Can you work these out from the model? Positions are in its coordinate system, mm. Face numbers are marked on the shaded views. A direction names the side the tool comes from. Give positions to 0.01 mm unless a question says otherwise; leave off trailing zeros. Write each loop counter-clockwise with the first axis right and the second up, starting at its lowest first coordinate (ties: lowest second). Pieces come first, ordered by that corner, then holes. Notation, with made-up numbers: M -5.5,42 L 34.5,42 A21 ccw 34.5,71 Z; hole C 35.25,70.5 d7. An arc over 180 degrees is marked long. Write each question's results on one line, items separated by ' | '.
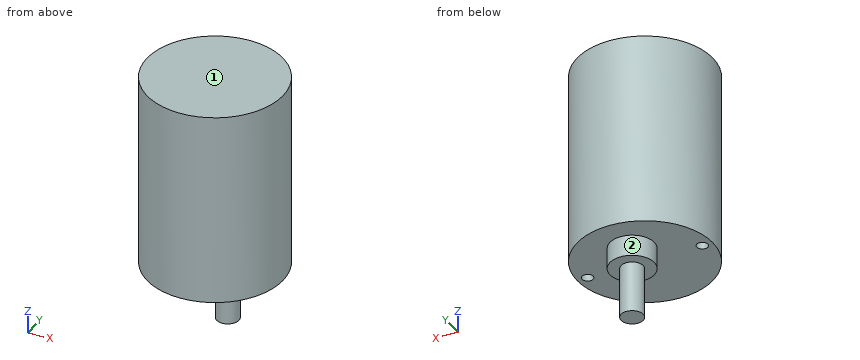
from build123d import *

# Parameters (mm, degrees)
SKETCH_1_R          = 18.35
EXTRUDE_1_DEPTH     = 52.4
SKETCH_1_4_R        = 6
EXTRUDE_2_DEPTH     = 5.7
SKETCH_1_5_R        = 3
EXTRUDE_3_DEPTH     = 19.5
SKETCH_1_6_R        = 1.5
CUT_EXTRUDE_1_DEPTH = 3


with BuildPart() as part:
    # 草图1 → 凸台-拉伸1 (new body)
    with BuildSketch(Plane.XY):
        Circle(SKETCH_1_R)
    extrude(amount=EXTRUDE_1_DEPTH)

    # 草图1<4> → 凸台-拉伸2 (add)
    with BuildSketch(Plane.XY):
        with Locations((0, 6.65)):
            Circle(SKETCH_1_4_R)
    extrude(amount=-EXTRUDE_2_DEPTH)

    # 草图1<5> → 凸台-拉伸3 (add)
    with BuildSketch(Plane.XY):
        with Locations((0, 6.65)):
            Circle(SKETCH_1_5_R)
    extrude(amount=-EXTRUDE_3_DEPTH)

    # 草图1<6> → 切除-拉伸1 (cut)
    with BuildSketch(Plane.XY):
        with Locations((-15.5, 0)):
            Circle(SKETCH_1_6_R)
        with Locations((15.5, 0)):
            Circle(SKETCH_1_6_R)
    extrude(amount=CUT_EXTRUDE_1_DEPTH, mode=Mode.SUBTRACT)


solid = part.part
Item 1: I want a section at B-B, the plane y = 4.5. Please give me the cut outline in (x, z), and give its area (3 significant figures).
Geometry says:
outline: M -17.79,0 L -5.6,0 L -5.6,-5.7 L -2.09,-5.7 L -2.09,-19.5 L 2.09,-19.5 L 2.09,-5.7 L 5.6,-5.7 L 5.6,0 L 17.79,0 L 17.79,52.4 L -17.79,52.4 Z | area: 1,990 mm2
Item 2: If I drill on line 1 (Z direction, x = 3.5, y = 8); line 2 (Z direction, x = -14, y = 8); line 3 (Y direction, x = 15.5, z = 1.9), over which ranges is the centre line in solid material (lowest first)? Write a range as from..to.
Geometry says:
line 1: z = -5.7..52.4 | line 2: z = 0..52.4 | line 3: y = -9.82..-1.5, 1.5..9.82
Item 3: For the marked faces 1 and 2, which set-ups out of +Z, -Z, +X, -X, +Y, -Y let a thin tool reach every point of the face, with its end or its side?
Geometry says:
face 1: +Z, +X, -X, +Y, -Y | face 2: -Z
Item 4: I want a section at D-D, the plane x = 16. Please give me the cut outline in (y, z), and give its area (3 significant figures).
Geometry says:
outline: M -8.98,0 L -1.41,0 L -1.41,3 L 1.41,3 L 1.41,0 L 8.98,0 L 8.98,52.4 L -8.98,52.4 Z | area: 933 mm2
Item 5: I want a section at C-C, the plane z = 17.5. Please give me the cut outline in (x, y).
Geometry says:
outline: C 0,0 d36.7
Item 6: I want a section at A-A, the plane x = 0. Please give me the cut outline in (y, z).
Geometry says:
outline: M -18.35,0 L 0.65,0 L 0.65,-5.7 L 3.65,-5.7 L 3.65,-19.5 L 9.65,-19.5 L 9.65,-5.7 L 12.65,-5.7 L 12.65,0 L 18.35,0 L 18.35,52.4 L -18.35,52.4 Z
Item 7: I'm going to push flat-ended pins straight in: pin 1 (10 mm diameter, centred on x = 13.5, y = -0.5, fed in from -Z); pin 2 (2 mm diameter, centred on x = 5, z = 18, fed in from +Y); pin 3 (1.5 mm diameter, centred on x = -15.5, y = -0.5, fed in from -Z). Where does each tip first touch, or does it pass through?
Geometry says:
pin 1: stops at z = 0 | pin 2: stops at y = 17.91 | pin 3: stops at z = 3
